Check sheet for the drawn part. Datum: minimum x, y, z corner. Units: mm. A direction names the side the tool comes from. Round coordinates to 2 decimals unless told otherwise and drop trailing zeros. Order: outer loops, then holes, each group sorted by start corner. A loop starts at its lowest first (then second) coordinate and runs counter-clockwise, first axis right, second up. Notation, with made-up numbers: M 13.5,-26 L 50.5,-26 A19 cw 50.5,3 Z; hole C -24,22 d9. An arc over 180 degrees is marked long. Use one line per item in the form item = value. Start each with the question number.
Item 1: Thickness scan on probe 1 along Z at (x, y) = (1.05, 6.25) (1 decimal); probe 2 along Z at (x, y) = (2.3, 14); probe 3 along Y at (x, z) = (1.05, 3.25) (1 decimal). Record the ranges inside material, lowest first. Write a range as [from, to].
Item 2: Cross-section at C-C on x = 4.05. Enter the section's corners in (y, z) (1 decimal).
Item 3: Cross-section at A-A on x = 1.45. Enter the section's corners in (y, z) (1 decimal).
Item 4: Cross-section at D-D on z = 12.5. Enter the section's corners in (x, y).
Item 5: Go/stop test with a flat-tipped pin: pin 1 Ø3.5 at (y, z) = (13.17, 16.04) entering from +X. Record where the tip stops, or that it passes through.
Item 6: Cross-section at B-B on y = 17.75. Enter the section's corners in (x, z).
Item 7: Tool access check on the marked faces 1 and 2. Record the directions out of +Z, -Z, +X, -X, +Y, -Y that give a thin tool (end or side, any length) a straight path to the whole face; none if there is none.
Item 8: Release check for a two-part mould opening along Y. For the marked faces 3, 4 and 5 record: +Y half, -Y half, draft (parallel to the pull), parting line (faces both ways), or undercut.
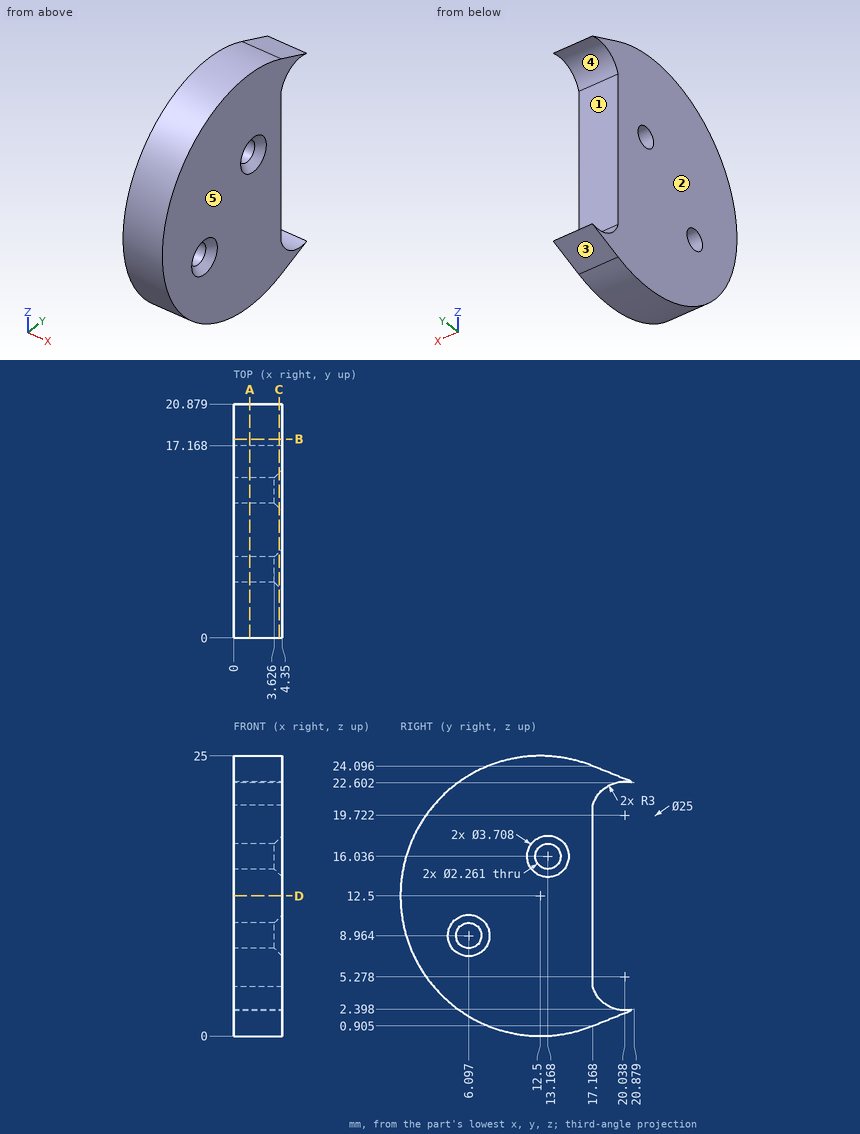
Output values:
q1.probe_1 = [1.7, 7.8], [10.1, 23.3]
q1.probe_2 = [0.09, 15.27], [16.8, 24.91]
q1.probe_3 = [4.1, 17.8]
q2.outline = M 17.2,0.9 L 20.9,2.4 A3 cw 17.2,4.4 L 17.2,20.6 A3 cw 20.9,22.6 L 17.2,24.1 A12.5 ccw long Z; hole C 6.1,9 d3.1; hole C 13.2,16 d3.1
q3.outline = M 17.2,0.9 L 20.9,2.4 A3 cw 17.2,4.4 L 17.2,20.6 A3 cw 20.9,22.6 L 17.2,24.1 A12.5 ccw long Z; hole C 6.1,9 d2.3; hole C 13.2,16 d2.3
q4.outline = M 0,0 L 4.35,0 L 4.35,17.17 L 0,17.17 Z
q5.pin_1 = 4.25
q6.outline = M 0,1.14 L 4.35,1.14 L 4.35,3.34 L 0,3.34 Z; M 0,21.66 L 4.35,21.66 L 4.35,23.86 L 0,23.86 Z
q7.face_1 = +X, -X, +Y
q7.face_2 = +Z, -Z, -X, +Y, -Y
q8.face_3 = +Y half
q8.face_4 = undercut
q8.face_5 = draft
